```python
from build123d import *

# Parameters (mm, degrees)
SKETCH2_R               = 3.2
BOSS_EXTRUDE1_DEPTH     = 2.6
CUT_EXTRUDE1_DEPTH      = 3
CUT_EXTRUDE1_DEPTH_BACK = 3


with BuildPart() as part:
    # Sketch1 → Revolve1 (revolve)
    with BuildSketch(Plane(origin=(0, 0, 0), x_dir=(0, 0, -1), z_dir=(1, 0, 0)), mode=Mode.PRIVATE) as revolve1_sk:
        Polygon((-11.5, 0), (-11.5, 3), (-10.00428681, 3), (-10.00428681, 3.777777778), (-8.703281017, 3.777777778), (-8.703281017, 4.555555556), (-7.548361646, 4.555555556), (-7.548361646, 5.333333333), (-6.509180682, 5.333333333), (-6.509180682, 6.111111111), (-5.565268632, 6.111111111), (-5.565268632, 6.888888889), (-4.702037743, 6.888888889), (-4.702037743, 7.666666667), (-3.908655746, 7.666666667), (-3.908655746, 8.444444444), (-3.176819128, 8.444444444), (-3.176819128, 9.222222222), (-2.5, 9.222222222), (-2.5, 10), (0, 10), (0, 0), align=None)
    revolve(revolve1_sk.sketch.rotate(Axis((0, 0, 0), (0, 1, 0)), 180), axis=Axis((0, 0, 0), (0, 1, 0)))

    # Sketch2 → Boss-Extrude1 (add)
    with BuildSketch(Plane.XZ):
        with Locations(Location((0, 0, 0), (0, 0, 270))):
            Circle(SKETCH2_R)
    extrude(amount=BOSS_EXTRUDE1_DEPTH)

    # Sketch2_3 → Cut-Extrude1 (cut, two sides: drawn at the far end of the back side and taken through both)
    with BuildSketch(Plane.XZ.offset(-CUT_EXTRUDE1_DEPTH_BACK)):
        with BuildLine():
            Line((-1.449137675, 1.45), (1.449137675, 1.45))
            ThreePointArc((1.449137675, 1.45), (0, -2.05), (-1.449137675, 1.45))
        make_face()
    extrude(amount=CUT_EXTRUDE1_DEPTH + CUT_EXTRUDE1_DEPTH_BACK, mode=Mode.SUBTRACT)


solid = part.part
```
Verification items for the finished model (mm, model axes). A direction names the side the tool comes from. Give positions to 0.01 mm unless a question says otherwise; leave off trailing zeros. Write each loop counter-clockwise with the first axis right and the second up, starting at its lowest first coordinate (ties: lowest second). Pieces come first, ordered by that corner, then holes. Notation, with made-up numbers: (77, 70.25) - (81, 70.25) arc R27 cw to (81, 94.25) - close; hole circle Ø4 at (-26, -6). An arc over 180 degrees is marked (long way). Put each result on its own line as item: value.
Q1. Depth check by flat-ended pin: P1, Ø7, axis at x = -4, z = 5.5, coming from the +Y side; P2, Ø1.8, axis at x = -0.5, z = -0.5, coming from the -Y side; P3, Ø3, axis at y = 3.5, z = -4, coming from the -X side. Enter the tip coordinate at first touch or a pass-through.
Result:
P1: y = 8.44
P2: y = 3
P3: x = -11.21
Q2. Section check C-C on y = -1.5. Record the cut outline in (x, z).
Result:
outline: circle Ø6.4 at (0, 0); hole (-1.45, 1.45) arc R2.05 ccw (long way) to (1.45, 1.45) - close
Q3. Scan lines: probe 1 along X at (y, z) = (0.65, 0); probe 2 along X at (y, z) = (-0.55, 0); probe 3 along Y at (x, z) = (10.5, 4). Record each from-to range of solid material in increasing order. Write a range as from..to.
Result:
probe 1: -11.5..-2.05, 2.05..11.5
probe 2: -3.2..-2.05, 2.05..3.2
probe 3: 0..3
Q4. Section check A-A on y = 1.25. Record the cut outline in (x, z).
Result:
outline: circle Ø23 at (0, 0); hole (-1.45, 1.45) arc R2.05 ccw (long way) to (1.45, 1.45) - close
Q5. Section check B-B on y = 8.75. Record the cut outline in (x, z), and give its area (3 significant figures).
Result:
outline: circle Ø6.35 at (0, 0)
area: 31.7 mm2
Q6. Mould release check, pull along Z, two halves, no side actions. Record for faces 1 (the face through (-8, 4.556, 0)), 2 (the face through (0, 3, 0)), 3 (the face through (9.766, 3.394, 2.169)): released by +Z, released by -Z, zero draft, split by the parting line, or undercut.
Result:
face 1: zero draft
face 2: undercut
face 3: split by the parting line
Q7. Set-up check for faces 4 (the face through (0.07, 0.24, -2.05)), 5 (the face through (-0.1, 9.6, 2.5)): record each of +Z, -Z, +X, -X, +Y, -Y from which the full face is reachable in a straight line by a thin tool's end or side.
Result:
face 4: -Y
face 5: +Y
